from build123d import *

# Parameters (mm, degrees)
BRIDA_BASE1_DEPTH             = 4
PLIEGUE_START                 = -21.07192
PLIEGUE_CROQUIZADO1_OUTLINE_W = 400
PLIEGUE_CROQUIZADO1_OUTLINE_H = 4
PLIEGUE_CROQUIZADO1_DEPTH     = 73.82192
PLIEGUE_START_2               = -24.25
PLIEGUE_CROQUIZADO1_2_DEPTH   = 0.02192
PLIEGUE_START_3               = -28.25
PLIEGUE_CROQUIZADO1_3_DEPTH   = 8
PLIEGUE_START_4               = -200
PLIEGUE_CROQUIZADO1_4_DEPTH   = 400
CROQUIS8_R                    = 7
CORTAR_EXTRUIR2_DEPTH         = 10
CORTAR_EXTRUIR3_REACH         = 218.197
CROQUIS9_R                    = 2.5


with BuildPart() as part:
    # Brida base1: sheet metal written as solids
    # Croquis1 → Brida base1 (new body)
    with BuildSketch(Plane(origin=(0, 0, 0), x_dir=(1, 0, 0), z_dir=(0, 1, 0))):
        with BuildLine():
            Line((170, -52.75), (190, -52.75))
            ThreePointArc((190, -52.75), (197.071067812, -49.821067812), (200, -42.75))
            Line((200, -42.75), (200, 42.75))
            ThreePointArc((200, 42.75), (197.071067812, 49.821067812), (190, 52.75))
            Line((190, 52.75), (-190, 52.75))
            ThreePointArc((-190, 52.75), (-197.071067812, 49.821067812), (-200, 42.75))
            Line((-200, 42.75), (-200, -42.75))
            ThreePointArc((-200, -42.75), (-197.071067812, -49.821067812), (-190, -52.75))
            Line((-190, -52.75), (-170, -52.75))
            ThreePointArc((-170, -52.75), (-162.928932188, -49.821067812), (-160, -42.75))
            Line((-160, -42.75), (-160, 7.25))
            ThreePointArc((-160, 7.25), (-157.071067812, 14.321067812), (-150, 17.25))
            Line((-150, 17.25), (150, 17.25))
            ThreePointArc((150, 17.25), (157.071067812, 14.321067812), (160, 7.25))
            Line((160, 7.25), (160, -42.75))
            ThreePointArc((160, -42.75), (162.928932188, -49.821067812), (170, -52.75))
        make_face()
    extrude(amount=-BRIDA_BASE1_DEPTH)

    # Pliegue croquizado1: read off the stored shape, not the designer's step
    # Pliegue croquizado1 outline → Pliegue croquizado1 (cut)
    with BuildSketch(Plane.XY.offset(PLIEGUE_START)):
        with Locations((0, -2)):
            Rectangle(PLIEGUE_CROQUIZADO1_OUTLINE_W, PLIEGUE_CROQUIZADO1_OUTLINE_H)
    extrude(amount=PLIEGUE_CROQUIZADO1_DEPTH, mode=Mode.SUBTRACT)

    # Pliegue croquizado1 2 outline → Pliegue croquizado1 2 (add)
    with BuildSketch(Plane.XY.offset(PLIEGUE_START_2)):
        with BuildLine():
            ThreePointArc((-190, 76.999999998), (-197.071067812, 74.07106781), (-200, 66.999999998))
            Line((-200, 66.999999998), (-200, 0))
            Line((-200, 0), (200, 0))
            Line((200, 0), (200, 66.999999998))
            ThreePointArc((200, 66.999999998), (197.071067812, 74.07106781), (190, 76.999999998))
            Line((190, 76.999999998), (170, 76.999999998))
            ThreePointArc((170, 76.999999998), (162.928932188, 74.07106781), (160, 66.999999998))
            Line((160, 66.999999998), (160, 16.999999998))
            ThreePointArc((160, 16.999999998), (157.071067812, 9.928932186), (150, 6.999999998))
            Line((150, 6.999999998), (-150, 6.999999998))
            ThreePointArc((-150, 6.999999998), (-157.071067812, 9.928932186), (-160, 16.999999998))
            Line((-160, 16.999999998), (-160, 66.999999998))
            ThreePointArc((-160, 66.999999998), (-162.928932188, 74.07106781), (-170, 76.999999998))
            Line((-170, 76.999999998), (-190, 76.999999998))
        make_face()
    extrude(amount=PLIEGUE_CROQUIZADO1_2_DEPTH)

    # Pliegue croquizado1 3 outline → Pliegue croquizado1 3 (add)
    with BuildSketch(Plane.XY.offset(PLIEGUE_START_3)):
        with BuildLine():
            ThreePointArc((-190, 76.999999998), (-197.071067812, 74.07106781), (-200, 66.999999998))
            Line((-200, 66.999999998), (-200, 0))
            Line((-200, 0), (200, 0))
            Line((200, 0), (200, 66.999999998))
            ThreePointArc((200, 66.999999998), (197.071067812, 74.07106781), (190, 76.999999998))
            Line((190, 76.999999998), (170, 76.999999998))
            ThreePointArc((170, 76.999999998), (162.928932188, 74.07106781), (160, 66.999999998))
            Line((160, 66.999999998), (160, 16.999999998))
            ThreePointArc((160, 16.999999998), (157.071067812, 9.928932186), (150, 6.999999998))
            Line((150, 6.999999998), (-150, 6.999999998))
            ThreePointArc((-150, 6.999999998), (-157.071067812, 9.928932186), (-160, 16.999999998))
            Line((-160, 16.999999998), (-160, 66.999999998))
            ThreePointArc((-160, 66.999999998), (-162.928932188, 74.07106781), (-170, 76.999999998))
            Line((-170, 76.999999998), (-190, 76.999999998))
        make_face()
    extrude(amount=PLIEGUE_CROQUIZADO1_3_DEPTH)

    # Pliegue croquizado1 4 outline → Pliegue croquizado1 4 (cut)
    with BuildSketch(Plane.YZ.offset(PLIEGUE_START_4)):
        with BuildLine():
            ThreePointArc((-4, -28.25), (-1.656854249, -22.593145751), (4, -20.25))
            Line((4, -20.25), (0, -20.25))
            Line((0, -20.25), (0, -21.07192))
            Line((0, -21.07192), (-4, -21.07192))
            Line((-4, -21.07192), (-4, -28.25))
        make_face()
        with BuildLine():
            ThreePointArc((4, -24.25), (1.171572875, -25.421572875), (0, -28.25))
            Line((0, -28.25), (76.999999998, -28.25))
            Line((76.999999998, -28.25), (76.999999998, -24.25))
            Line((76.999999998, -24.25), (4, -24.25))
        make_face()
    extrude(amount=PLIEGUE_CROQUIZADO1_4_DEPTH, mode=Mode.SUBTRACT)

    # Croquis8 → Cortar-Extruir2 (cut)
    with BuildSketch(Plane(origin=(0, 0, 0), x_dir=(1, 0, 0), z_dir=(0, 1, 0))):
        with Locations(Location((0, 37.75, 0), (0, 0, 270))):
            Circle(CROQUIS8_R)
    extrude(amount=-CORTAR_EXTRUIR2_DEPTH, mode=Mode.SUBTRACT)

    # Croquis9 → Cortar-Extruir3 (cut, up to next)
    with BuildSketch(Plane(origin=(0, 0, -24.25), x_dir=(-1, 0, 0), z_dir=(0, 0, -1)), mode=Mode.PRIVATE) as cortar_extruir3_sk1:
        with Locations(Location((180, 11.999999998, 0), (0, 0, 90))):
            Circle(CROQUIS9_R)
    cortar_extruir3_tool1 = extrude(cortar_extruir3_sk1.sketch, amount=-CORTAR_EXTRUIR3_REACH, mode=Mode.PRIVATE) & part.part
    # Croquis9 → Cortar-Extruir3 (cut, up to next)
    with BuildSketch(Plane(origin=(0, 0, -24.25), x_dir=(-1, 0, 0), z_dir=(0, 0, -1)), mode=Mode.PRIVATE) as cortar_extruir3_sk2:
        with Locations(Location((180, 66.999999998, 0), (0, 0, 90))):
            Circle(CROQUIS9_R)
    cortar_extruir3_tool2 = extrude(cortar_extruir3_sk2.sketch, amount=-CORTAR_EXTRUIR3_REACH, mode=Mode.PRIVATE) & part.part
    # Croquis9 → Cortar-Extruir3 (cut, up to next)
    with BuildSketch(Plane(origin=(0, 0, -24.25), x_dir=(-1, 0, 0), z_dir=(0, 0, -1)), mode=Mode.PRIVATE) as cortar_extruir3_sk3:
        with Locations(Location((170, 51.999999998, 0), (0, 0, 90))):
            Circle(CROQUIS9_R)
    cortar_extruir3_tool3 = extrude(cortar_extruir3_sk3.sketch, amount=-CORTAR_EXTRUIR3_REACH, mode=Mode.PRIVATE) & part.part
    # Croquis9 → Cortar-Extruir3 (cut, up to next)
    with BuildSketch(Plane(origin=(0, 0, -24.25), x_dir=(-1, 0, 0), z_dir=(0, 0, -1)), mode=Mode.PRIVATE) as cortar_extruir3_sk4:
        with Locations(Location((190, 51.999999998, 0), (0, 0, 90))):
            Circle(CROQUIS9_R)
    cortar_extruir3_tool4 = extrude(cortar_extruir3_sk4.sketch, amount=-CORTAR_EXTRUIR3_REACH, mode=Mode.PRIVATE) & part.part
    # Croquis9 → Cortar-Extruir3 (cut, up to next)
    with BuildSketch(Plane(origin=(0, 0, -24.25), x_dir=(-1, 0, 0), z_dir=(0, 0, -1)), mode=Mode.PRIVATE) as cortar_extruir3_sk5:
        with Locations(Location((180, 36.999999998, 0), (0, 0, 90))):
            Circle(CROQUIS9_R)
    cortar_extruir3_tool5 = extrude(cortar_extruir3_sk5.sketch, amount=-CORTAR_EXTRUIR3_REACH, mode=Mode.PRIVATE) & part.part
    # Croquis9 → Cortar-Extruir3 (cut, up to next)
    with BuildSketch(Plane(origin=(0, 0, -24.25), x_dir=(-1, 0, 0), z_dir=(0, 0, -1)), mode=Mode.PRIVATE) as cortar_extruir3_sk6:
        with Locations(Location((170, 21.999999998, 0), (0, 0, 90))):
            Circle(CROQUIS9_R)
    cortar_extruir3_tool6 = extrude(cortar_extruir3_sk6.sketch, amount=-CORTAR_EXTRUIR3_REACH, mode=Mode.PRIVATE) & part.part
    # Croquis9 → Cortar-Extruir3 (cut, up to next)
    with BuildSketch(Plane(origin=(0, 0, -24.25), x_dir=(-1, 0, 0), z_dir=(0, 0, -1)), mode=Mode.PRIVATE) as cortar_extruir3_sk7:
        with Locations(Location((190, 21.999999998, 0), (0, 0, 90))):
            Circle(CROQUIS9_R)
    cortar_extruir3_tool7 = extrude(cortar_extruir3_sk7.sketch, amount=-CORTAR_EXTRUIR3_REACH, mode=Mode.PRIVATE) & part.part
    # Croquis9 → Cortar-Extruir3 (cut, up to next)
    with BuildSketch(Plane(origin=(0, 0, -24.25), x_dir=(-1, 0, 0), z_dir=(0, 0, -1)), mode=Mode.PRIVATE) as cortar_extruir3_sk8:
        with Locations(Location((-190, 21.999999998, 0), (0, 0, 90))):
            Circle(CROQUIS9_R)
    cortar_extruir3_tool8 = extrude(cortar_extruir3_sk8.sketch, amount=-CORTAR_EXTRUIR3_REACH, mode=Mode.PRIVATE) & part.part
    # Croquis9 → Cortar-Extruir3 (cut, up to next)
    with BuildSketch(Plane(origin=(0, 0, -24.25), x_dir=(-1, 0, 0), z_dir=(0, 0, -1)), mode=Mode.PRIVATE) as cortar_extruir3_sk9:
        with Locations(Location((-170, 21.999999998, 0), (0, 0, 90))):
            Circle(CROQUIS9_R)
    cortar_extruir3_tool9 = extrude(cortar_extruir3_sk9.sketch, amount=-CORTAR_EXTRUIR3_REACH, mode=Mode.PRIVATE) & part.part
    # Croquis9 → Cortar-Extruir3 (cut, up to next)
    with BuildSketch(Plane(origin=(0, 0, -24.25), x_dir=(-1, 0, 0), z_dir=(0, 0, -1)), mode=Mode.PRIVATE) as cortar_extruir3_sk10:
        with Locations(Location((-180, 36.999999998, 0), (0, 0, 90))):
            Circle(CROQUIS9_R)
    cortar_extruir3_tool10 = extrude(cortar_extruir3_sk10.sketch, amount=-CORTAR_EXTRUIR3_REACH, mode=Mode.PRIVATE) & part.part
    # Croquis9 → Cortar-Extruir3 (cut, up to next)
    with BuildSketch(Plane(origin=(0, 0, -24.25), x_dir=(-1, 0, 0), z_dir=(0, 0, -1)), mode=Mode.PRIVATE) as cortar_extruir3_sk11:
        with Locations(Location((-190, 51.999999998, 0), (0, 0, 90))):
            Circle(CROQUIS9_R)
    cortar_extruir3_tool11 = extrude(cortar_extruir3_sk11.sketch, amount=-CORTAR_EXTRUIR3_REACH, mode=Mode.PRIVATE) & part.part
    # Croquis9 → Cortar-Extruir3 (cut, up to next)
    with BuildSketch(Plane(origin=(0, 0, -24.25), x_dir=(-1, 0, 0), z_dir=(0, 0, -1)), mode=Mode.PRIVATE) as cortar_extruir3_sk12:
        with Locations(Location((-170, 51.999999998, 0), (0, 0, 90))):
            Circle(CROQUIS9_R)
    cortar_extruir3_tool12 = extrude(cortar_extruir3_sk12.sketch, amount=-CORTAR_EXTRUIR3_REACH, mode=Mode.PRIVATE) & part.part
    # Croquis9 → Cortar-Extruir3 (cut, up to next)
    with BuildSketch(Plane(origin=(0, 0, -24.25), x_dir=(-1, 0, 0), z_dir=(0, 0, -1)), mode=Mode.PRIVATE) as cortar_extruir3_sk13:
        with Locations(Location((-180, 66.999999998, 0), (0, 0, 90))):
            Circle(CROQUIS9_R)
    cortar_extruir3_tool13 = extrude(cortar_extruir3_sk13.sketch, amount=-CORTAR_EXTRUIR3_REACH, mode=Mode.PRIVATE) & part.part
    # Croquis9 → Cortar-Extruir3 (cut, up to next)
    with BuildSketch(Plane(origin=(0, 0, -24.25), x_dir=(-1, 0, 0), z_dir=(0, 0, -1)), mode=Mode.PRIVATE) as cortar_extruir3_sk14:
        with Locations(Location((-180, 11.999999998, 0), (0, 0, 90))):
            Circle(CROQUIS9_R)
    cortar_extruir3_tool14 = extrude(cortar_extruir3_sk14.sketch, amount=-CORTAR_EXTRUIR3_REACH, mode=Mode.PRIVATE) & part.part
    add(cortar_extruir3_tool1.solids().sort_by_distance((-180, 12, -24.25))[0], mode=Mode.SUBTRACT)
    add(cortar_extruir3_tool2.solids().sort_by_distance((-180, 67, -24.25))[0], mode=Mode.SUBTRACT)
    add(cortar_extruir3_tool3.solids().sort_by_distance((-170, 52, -24.25))[0], mode=Mode.SUBTRACT)
    add(cortar_extruir3_tool4.solids().sort_by_distance((-190, 52, -24.25))[0], mode=Mode.SUBTRACT)
    add(cortar_extruir3_tool5.solids().sort_by_distance((-180, 37, -24.25))[0], mode=Mode.SUBTRACT)
    add(cortar_extruir3_tool6.solids().sort_by_distance((-170, 22, -24.25))[0], mode=Mode.SUBTRACT)
    add(cortar_extruir3_tool7.solids().sort_by_distance((-190, 22, -24.25))[0], mode=Mode.SUBTRACT)
    add(cortar_extruir3_tool8.solids().sort_by_distance((190, 22, -24.25))[0], mode=Mode.SUBTRACT)
    add(cortar_extruir3_tool9.solids().sort_by_distance((170, 22, -24.25))[0], mode=Mode.SUBTRACT)
    add(cortar_extruir3_tool10.solids().sort_by_distance((180, 37, -24.25))[0], mode=Mode.SUBTRACT)
    add(cortar_extruir3_tool11.solids().sort_by_distance((190, 52, -24.25))[0], mode=Mode.SUBTRACT)
    add(cortar_extruir3_tool12.solids().sort_by_distance((170, 52, -24.25))[0], mode=Mode.SUBTRACT)
    add(cortar_extruir3_tool13.solids().sort_by_distance((180, 67, -24.25))[0], mode=Mode.SUBTRACT)
    add(cortar_extruir3_tool14.solids().sort_by_distance((180, 12, -24.25))[0], mode=Mode.SUBTRACT)


solid = part.part
Verification items for the finished model (mm, model axes). A direction names the side the tool comes from. Coordinates: 2 decimals unless noted, no trailing zeros. Order: outer loops, then holes, each group sorted by start corner. A loop starts at its lowest first (then second) coordinate and runs counter-clockwise, first axis right, second up. Notation, with made-up numbers: M -16.75,17 L 33.25,17 A12 ccw 33.25,37 Z; hole C 7,41 d6. An arc over 180 degrees is marked long. One line per item, written item: value. Start each with the question number.
Item 1: Mould release check, pull along X, two halves, no side actions. Record for faces 1 (the flat face through (-200, 26, -24)), 2 (the cylindrical face through (197.15, 73.99, -22.28)), 3 (the cylindrical face through (-162.85, 73.99, -22.28)): released by +X, released by -X, zero draft, split by the parting line, or undercut.
Item 2: Sectioned sample at B-B (x = -71). Enter the section's corners in (y, z), then the cut area to 3 significant figures.
Item 3: Access from +Z, -Z, +X, -X, +Y, -Y to the whole of each face (thin tool, end or side, straight path). Record for faces 4 (the flat face through (-16, 6, -24.25)), 5 (the cylindrical face through (-196.99, -1.97, -49.9)), 6 (the cylindrical face through (-156.99, 9.85, -22.28)).
Item 4: Sectioned sample at A-A (x = 0). Enter the section's corners in (y, z).
Item 5: Gauge pin test, flat ends, axial feed: pin 1 (8 mm diameter, centred on x = -190, y = 22, fed in from -Z); pin 2 (2 mm diameter, centred on x = -28, z = -37.5, fed in from +Y); pin 3 (1.5 mm diameter, centred on x = -45, z = -26.5, fed in from -Y). Record the tip position at first contact, or that the pin passes through.
Item 6: Scan lines: probe 1 along X at (y, z) = (52, -22.15); probe 2 along X at (y, z) = (37, -21.65); probe 3 along X at (y, z) = (12, -21). Record each from-to range of solid material in increasing order.
Conclusion:
1. face 1: released by -X
1. face 2: released by +X
1. face 3: undercut
2. outline: M -4,-52.75 L 0,-52.75 L 0,-28.25 A4 cw 4,-24.25 L 7,-24.25 L 7,-20.25 L 4,-20.25 A8 ccw -4,-28.25 Z
2. area: 148 mm^2
3. face 4: -Z, +X, -X, +Y
3. face 5: -Z, -X, +Y, -Y
3. face 6: +Z, -Z, +Y
4. outline: M -4,-52.75 L 0,-52.75 L 0,-44.75 L -4,-44.75 Z; M -4,-30.75 L 0,-30.75 L 0,-28.25 A4 cw 4,-24.25 L 7,-24.25 L 7,-20.25 L 4,-20.25 A8 ccw -4,-28.25 Z
5. pin 1: stops at z = -24.25
5. pin 2: stops at y = 0
5. pin 3: stops at y = -3.94
6. probe 1: x = -200 to -192.5, -187.5 to -172.5, -167.5 to -160, 160 to 167.5, 172.5 to 187.5, 192.5 to 200
6. probe 2: x = -200 to -182.5, -177.5 to -160, 160 to 177.5, 182.5 to 200
6. probe 3: x = -200 to -182.5, -177.5 to -158.66, 158.66 to 177.5, 182.5 to 200
